from build123d import *

# Parameters (mm, degrees)
F1_DEPTH      = 50
F1_DEPTH_BACK = 50
F2_T1_DEPTH   = 82.5
F2_T3_DEPTH   = 116.1726990145
F2_T5_DEPTH   = 11.25
F2_T10_DEPTH  = 79
F2_T15_DEPTH  = 128.4622783495
F2_T21_DEPTH  = 128.4622783495
F2_T25_DEPTH  = 79
F2_T32_DEPTH  = 122.4226990145
F2_T36_DEPTH  = 17.5


# Not quite as in the source:
# - a fillet or chamfer that OpenCascade refuses, or shapes differently, is made with other operations: its cross-section is extruded or revolved along the edge and cut away or added


with BuildPart() as f1:
    # F0 (on Top) → F1 (new body, two sides)
    with BuildSketch(Plane.XY) as f1_sk:
        Polygon((50, 35), (41.281031703, 35), (-48.7711521192, -28.0365286756), (-50, -26.281031703), (-51.638463841, -23.940369073), (-55.7346234436, -26.8076807948), (-52.8673117218, -30.9038403974), (-50, -35), (45, 31.5), (45, -35), (50, -35), align=None)
    extrude(amount=F1_DEPTH)
    extrude(f1_sk.sketch, amount=-F1_DEPTH_BACK)

    # F2: fillet of radius 2.5 on 5 edges, made by hand

    # F2_s2 → F2_t1 (cut)
    with BuildSketch(Plane.XZ.offset(-41.25)):
        with BuildLine():
            ThreePointArc((47.5, -50), (49.267766953, -49.267766953), (50, -47.5))
            Line((50, -47.5), (50, -50))
            Line((50, -50), (47.5, -50))
        make_face()
    extrude(amount=F2_T1_DEPTH, mode=Mode.SUBTRACT)

    # F2_s4 → F2_t3 (cut)
    with BuildSketch(Plane(origin=(49.2685429281, 34.4879800497, 0), x_dir=(0, 0, 1), z_dir=(-0.8192319205, -0.5734623444, 0))):
        with BuildLine():
            ThreePointArc((-50, 2.5), (-49.267766953, 4.267766953), (-47.5, 5))
            Line((-47.5, 5), (-50, 5))
            Line((-50, 5), (-50, 2.5))
        make_face()
    extrude(amount=F2_T3_DEPTH, mode=Mode.SUBTRACT)

    # F2_s6 → F2_t5 (cut)
    with BuildSketch(Plane(origin=(-2.8673117218, 4.0961596026, 0), x_dir=(0, 0, 1), z_dir=(-0.5734623444, 0.8192319205, 0))):
        with BuildLine():
            ThreePointArc((-50, -58.5327780787), (-49.267766953, -56.7650111257), (-47.5, -56.0327780787))
            Line((-47.5, -56.0327780787), (-50, -56.0327780787))
            Line((-50, -56.0327780787), (-50, -58.5327780787))
        make_face()
    extrude(amount=F2_T5_DEPTH, mode=Mode.SUBTRACT)


with BuildPart() as f2_tool8:
    # F2_s9 → F2_t10 (new body)
    with BuildSketch(Plane.XZ.offset(-37.75)):
        with BuildLine():
            ThreePointArc((47.5, -50), (45.732233047, -49.267766953), (45, -47.5))
            Line((45, -47.5), (45, -50))
            Line((45, -50), (47.5, -50))
        make_face()
    extrude(amount=F2_T10_DEPTH)

    split(bisect_by=Plane(origin=(0, 0, 0), x_dir=(0, 0, 1), z_dir=(0.5734623444, -0.8192319205, 0)), keep=Keep.TOP)


with BuildPart() as f1_1:
    add(f1.part)

    # F2_t7: cut F2_tool8
    add(f2_tool8.part, mode=Mode.SUBTRACT)


with BuildPart() as f2_tool13:
    # F2_s14 → F2_t15 (new body)
    with BuildSketch(Plane(origin=(-55.1201995032, -38.5841396523, 0), x_dir=(0, 0, 1), z_dir=(0.8192319205, 0.5734623444, 0))):
        with BuildLine():
            ThreePointArc((-47.5, 0), (-49.267766953, -0.732233047), (-50, -2.5))
            Line((-50, -2.5), (-50, 0))
            Line((-50, 0), (-47.5, 0))
        make_face()
    extrude(amount=F2_T15_DEPTH)

    split(bisect_by=Plane.YZ.offset(45), keep=Keep.BOTTOM)


with BuildPart() as f1_2:
    add(f1_1.part)

    # F2_t12: cut F2_tool13
    add(f2_tool13.part, mode=Mode.SUBTRACT)


with BuildPart() as f2_tool19:
    # F2_s20 → F2_t21 (new body)
    with BuildSketch(Plane(origin=(-55.1201995032, -38.5841396523, 0), x_dir=(0, 0, 1), z_dir=(0.8192319205, 0.5734623444, 0))):
        with BuildLine():
            ThreePointArc((-47.5, 0), (-49.267766953, -0.732233047), (-50, -2.5))
            Line((-50, -2.5), (-50, 0))
            Line((-50, 0), (-47.5, 0))
        make_face()
    extrude(amount=F2_T21_DEPTH)

    split(bisect_by=Plane.YZ.offset(45), keep=Keep.TOP)


with BuildPart() as f2_tool23:
    # F2_s24 → F2_t25 (new body)
    with BuildSketch(Plane.XZ.offset(-37.75)):
        with BuildLine():
            ThreePointArc((47.5, -50), (45.732233047, -49.267766953), (45, -47.5))
            Line((45, -47.5), (45, -50))
            Line((45, -50), (47.5, -50))
        make_face()
    extrude(amount=F2_T25_DEPTH)

    split(bisect_by=Plane(origin=(0, 0, 0), x_dir=(0, 0, 1), z_dir=(-0.5734623444, 0.8192319205, 0)), keep=Keep.TOP)


with BuildPart() as f2_tool19_1:
    add(f2_tool19.part)

    # F2_t27: intersect F2_tool23
    add(f2_tool23.part, mode=Mode.INTERSECT)


with BuildPart() as f1_3:
    add(f1_2.part)

    # F2_t17: cut F2_tool19
    add(f2_tool19_1.part, mode=Mode.SUBTRACT)


with BuildPart() as f2_tool30:
    # F2_s31 → F2_t32 (new body)
    with BuildSketch(Plane(origin=(49.2685429281, 34.4879800497, 0), x_dir=(0, 0, 1), z_dir=(-0.8192319205, -0.5734623444, 0))):
        with BuildLine():
            ThreePointArc((-50, 2.5), (-49.267766953, 4.267766953), (-47.5, 5))
            Line((-47.5, 5), (-50, 5))
            Line((-50, 5), (-50, 2.5))
        make_face()
    extrude(amount=F2_T32_DEPTH)

    split(bisect_by=Plane(origin=(-45.9038403974, -32.1326882782, 0), x_dir=(0, 0, 1), z_dir=(-0.8192319205, -0.5734623444, 0)), keep=Keep.TOP)


with BuildPart() as f2_tool34:
    # F2_s35 → F2_t36 (new body)
    with BuildSketch(Plane(origin=(0.7168279305, -1.0240399006, 0), x_dir=(0, 0, 1), z_dir=(-0.5734623444, 0.8192319205, 0))):
        with BuildLine():
            ThreePointArc((-50, -58.5327780787), (-49.267766953, -56.7650111257), (-47.5, -56.0327780787))
            Line((-47.5, -56.0327780787), (-50, -56.0327780787))
            Line((-50, -56.0327780787), (-50, -58.5327780787))
        make_face()
    extrude(amount=F2_T36_DEPTH)

    split(bisect_by=Plane(origin=(-2.8673117218, 4.0961596026, 0), x_dir=(0, 0, 1), z_dir=(0.5734623444, -0.8192319205, 0)), keep=Keep.TOP)


with BuildPart() as f2_tool30_1:
    add(f2_tool30.part)

    # F2_t38: intersect F2_tool34
    add(f2_tool34.part, mode=Mode.INTERSECT)


with BuildPart() as f1_4:
    add(f1_3.part)

    # F2_t28: cut F2_tool30
    add(f2_tool30_1.part, mode=Mode.SUBTRACT)


solid = f1_4.part
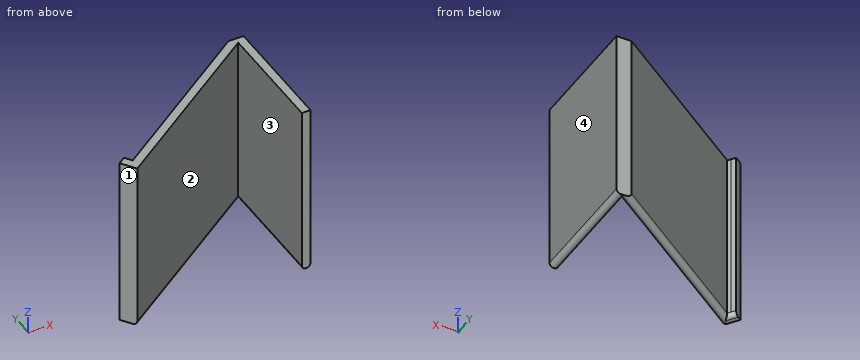
Check sheet for the modelled part. Datum: model origin and axes. Units: mm. Face numbers are marked on the shaded views. Round coordinates to 2 decimals unless told otherwise and drop trailing zeros. Order: outer loops, then holes, each group sorted by start corner. A loop starts at its lowest first (then second) coordinate and runs counter-clockwise, first axis right, second up.
(1) Go/stop test with flat-tipped pins: P1, Ø4, axis at x = 20, z = -3.5, coming from the -Y side; P2, Ø2, axis at x = 38, z = 20.5, coming from the -Y side; P3, Ø20, axis at y = -14, z = 22, coming from the -X side. Record where each tip stops, or that it passes through.
(2) Draft check along X on the marked faces 1, 2, 3 and 4. Enter one of: pulls with the +X half, pulls with the -X half, needs draft (parallel to the pull), parting line crosses it, or undercut.
(3) Scan lines: probe 1 along X at (y, z) = (6, 33.5); probe 2 along X at (y, z) = (-22.5, -2.5); probe 3 along X at (y, z) = (-25, 32). Record each from-to range of solid material in increasing order.
(4) Cross-section at A-A, the plane z = 0. Enter the section's corners in (x, y).
Check sheet entries:
1. P1: stops at y = 12.6
1. P2: stops at y = 25.9
1. P3: stops at x = -51.72
2. face 1: pulls with the -X half
2. face 2: undercut
2. face 3: undercut
2. face 4: pulls with the +X half
3. probe 1: x = -0.15 to 8.57, 45 to 50
3. probe 2: x = -40.86 to -32.14, 45 to 50
3. probe 3: x = -53.15 to -50.9, -44.43 to -35.71, 45 to 50
4. outline: (-55.73, -26.81) - (-50, -35) - (45, 31.5) - (45, -35) - (50, -35) - (50, 35) - (41.28, 35) - (-48.77, -28.04) - (-51.64, -23.94) - close
